Could you check a few things on this model? Use its own coordinates, in mm. Face numbers are marked on the shaded views. A direction names the side the tool comes from. Round coordinates to 2 decimals unless told otherwise and drop trailing zeros. Loops run counter-clockwise (first coordinate to the right, second up) from the corner with the lowest first, then second, coordinate; pieces in that order, holes last.
from build123d import *

# Parameters (mm, degrees)
REVOLVE1_ANGLE          = 180
CUT_EXTRUDE1_DEPTH      = 114.578166916
CUT_EXTRUDE1_DEPTH_BACK = 114.578166916
SKETCH3_R               = 9
FILLET1_R               = 2


with BuildPart() as part:
    # Sketch2 → Revolve1 (revolve)
    with BuildSketch(Plane(origin=(0, 0, 0), x_dir=(1, 0, 0), z_dir=(0, 1, 0))):
        Polygon((-5, 80), (0, 80), (0, 20), (-10, 20), (-10, 40), (-5, 40), align=None)
        Polygon((10, 20), (0, 20), (0, 80), (5, 80), (5, 40), (10, 40), align=None)
    revolve(axis=Axis((-0.5, 0, 0), (1, 0, 0)), revolution_arc=REVOLVE1_ANGLE)

    # Sketch3 → Cut-Extrude1 (cut, two sides: drawn at the far end of the back side and taken through both)
    with BuildSketch(Plane(origin=(0, 0, 0), x_dir=(0, 0, -1), z_dir=(1, 0, 0)).offset(-CUT_EXTRUDE1_DEPTH_BACK)):
        with Locations((-51.961524227, 30)):
            Circle(SKETCH3_R)
        with Locations((0, 60)):
            Circle(SKETCH3_R)
        with Locations((51.961524227, 30)):
            Circle(SKETCH3_R)
    extrude(amount=CUT_EXTRUDE1_DEPTH + CUT_EXTRUDE1_DEPTH_BACK, mode=Mode.SUBTRACT)

    # Fillet1
    fillet1_edges = [part.edges().sort_by_distance(p)[0] for p in [
        (5, 40, 0),
        (-5, 40, 0),
    ]]
    fillet(fillet1_edges, radius=FILLET1_R)


solid = part.part
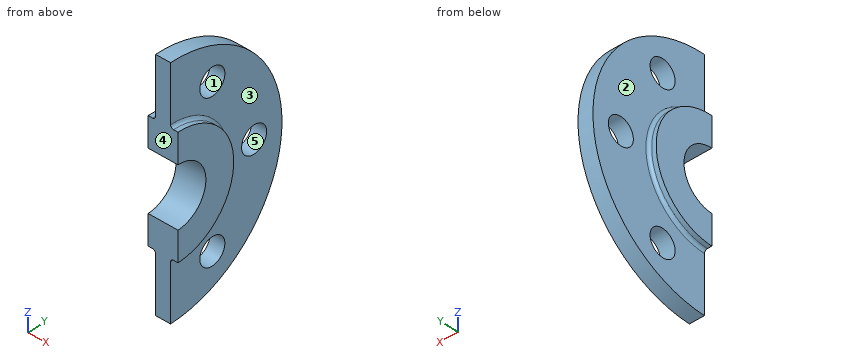
Item 1: If I drill on line 1 along Y through (x, z) = (-0.25, 0); line 2 along X through (y, z) = (69, -6); line 3 along Z through (x, y) = (0.5, 30), over which ranges is the centre line in solid material (lowest first)?
Results list:
line 1: y = 20 to 51, 69 to 80
line 2: x = -5 to 5
line 3: z = -74.16 to -60.96, -42.96 to 42.96, 60.96 to 74.16
Item 2: For the marked faces 1 and 2, which set-ups out of +Z, -Z, +X, -X, +Y, -Y let a thin tool reach every point of the face, with its end or its side?
Results list:
face 1: +X, -X
face 2: -X, +Y
Item 3: If we section it at B-B, the plane x = -2.75: Please give me the cut outline in (y, z).
Results list:
outline: (0, -80) arc R80 ccw to (0, 80) - (0, 20) arc R20 cw to (0, -20) - close; hole circle Ø18 at (30, -51.96); hole circle Ø18 at (30, 51.96); hole circle Ø18 at (60, 0)
Item 4: If we section it at A-A, the plane z = 0: Please give me the cut outline in (x, y), then the cut area to 3 significant figures.
Results list:
outline: (-10, 20) - (10, 20) - (10, 40) - (7, 40) arc R2 cw to (5, 42) - (5, 51) - (-5, 51) - (-5, 42) arc R2 cw to (-7, 40) - (-10, 40) - close; (-5, 69) - (5, 69) - (5, 80) - (-5, 80) - close
area: 622 mm2
Item 5: If we section it at C-C, the plane y = 60: Please give me the cut outline in (x, z).
Results list:
outline: (-5, -52.92) - (5, -52.92) - (5, -9) - (-5, -9) - close; (-5, 9) - (5, 9) - (5, 52.92) - (-5, 52.92) - close
Item 6: If we section it at D-D, the plane y = 48: Please give me the cut outline in (x, z).
Results list:
outline: (-5, -64) - (5, -64) - (5, 64) - (-5, 64) - close
Item 7: Will these pins go through, and if not, where does the flat tip stop? pin 1 (5 mm diameter, centred on x = 0, y = 53.5, fed in from +Z); pin 2 (8 mm diameter, centred on x = -4, z = -50, fed in from -Y); pin 3 (1.5 mm diameter, centred on x = 5.5, y = 19, fed in from +Z); pin 4 (23.5 mm diameter, centred on y = 30, z = -51.96, fed in from +X).
Results list:
pin 1: stops at z = 61.64
pin 2: stops at y = 0
pin 3: stops at z = 77.85
pin 4: stops at x = 5
Item 8: We'd pull the mould along Y, two halves only. Please class the marked faces 3, 4 and 5: released by +Y, released by -Y, zero draft, split by the parting line, or undercut.
Results list:
face 3: zero draft
face 4: released by -Y
face 5: undercut
